from build123d import *

# Parameters (mm, degrees)
SKETCH1_W           = 20.828
SKETCH1_H           = 40.386
BOSS_EXTRUDE1_DEPTH = 38.1
SKETCH2_W           = 20.828
SKETCH2_H           = 59.8424
SKETCH2_R           = 1.98755
BOSS_EXTRUDE2_DEPTH = 2.6162
SKETCH5_R           = 2.8575
BOSS_EXTRUDE3_DEPTH = 4.2418
CHAMFER1_SIZE       = 5.08
FILLET4_R           = 1.016


with BuildPart() as part:
    # Sketch1 → Boss-Extrude1 (new body)
    with BuildSketch(Plane(origin=(0, 0, 0), x_dir=(1, 0, 0), z_dir=(0, 1, 0))):
        with Locations((10.414, 20.193)):
            Rectangle(SKETCH1_W, SKETCH1_H)
    extrude(amount=BOSS_EXTRUDE1_DEPTH)

    # Sketch2 → Boss-Extrude2 (add)
    with BuildSketch(Plane(origin=(0, 27.7368, 0), x_dir=(1, 0, 0), z_dir=(0, 1, 0))):
        with Locations((10.414, 20.193)):
            Rectangle(SKETCH2_W, SKETCH2_H)
        with Locations((4.8641, 45.2501)):
            Circle(SKETCH2_R, mode=Mode.SUBTRACT)
        with Locations((15.9639, 45.2501)):
            Circle(SKETCH2_R, mode=Mode.SUBTRACT)
        with Locations((15.9639, -4.8641)):
            Circle(SKETCH2_R, mode=Mode.SUBTRACT)
        with Locations((4.8641, -4.8641)):
            Circle(SKETCH2_R, mode=Mode.SUBTRACT)
    extrude(amount=BOSS_EXTRUDE2_DEPTH)

    # Sketch4 → Revolve1 (revolve)
    with BuildSketch(Plane(origin=(10.414, 0, 0), x_dir=(0, 0, -1), z_dir=(1, 0, 0))):
        Polygon((30.3911, 40.259), (26.289, 40.259), (24.3078, 38.1), (30.3911, 38.1), align=None)
    revolve(axis=Axis((10.414, 40.259, -30.3911), (0, -1, 0)))

    # Sketch5 → Boss-Extrude3 (add)
    with BuildSketch(Plane(origin=(0, 40.259, 0), x_dir=(1, 0, 0), z_dir=(0, 1, 0))):
        with Locations((10.414, 30.3911)):
            Circle(SKETCH5_R)
    extrude(amount=BOSS_EXTRUDE3_DEPTH)

    # Chamfer1
    chamfer1_edges = [part.edges().sort_by_distance(p)[0] for p in [
        (10.414, 38.1, 0),
    ]]
    chamfer(chamfer1_edges, length=CHAMFER1_SIZE)

    # Fillet4
    fillet4_edges = [part.edges().sort_by_distance(p)[0] for p in [
        (10.414, 38.1, -40.386),
        (20.828, 38.1, -22.733),
        (0, 38.1, -22.733),
        (10.414, 38.1, -36.4744),
        (10.414, 38.1, -5.08),
        (20.828, 35.56, -2.54),
        (10.414, 33.02, 0),
        (0, 35.56, -2.54),
        (10.414, 0, -40.386),
        (0, 13.8684, -40.386),
        (0, 0, -20.193),
        (20.828, 0, -20.193),
        (10.414, 0, 0),
        (20.828, 13.8684, -40.386),
        (0, 13.8684, 0),
        (20.828, 13.8684, 0),
        (0, 34.2265, -40.386),
        (20.828, 34.2265, -40.386),
        (0, 29.0449, 9.7282),
        (20.828, 29.0449, 9.7282),
        (0, 29.0449, -50.1142),
        (20.828, 29.0449, -50.1142),
    ]]
    fillet(fillet4_edges, radius=FILLET4_R)


solid = part.part
Verification items for the finished model (mm, model axes). A direction names the side the tool comes from. Round coordinates to 2 decimals unless told otherwise and drop trailing zeros. Loops run counter-clockwise (first coordinate to the right, second up) from the corner with the lowest first, then second, coordinate; pieces in that order, holes last. Notation, with made-up numbers: (-31, 18) - (-14, 18) arc R23 cw to (-14, 41) - close; hole circle Ø6 at (-16, 68). An arc over 180 degrees is marked (long way). Answer in a Markdown table with one row per item. Add a question column.
Q1. Section check B-B on z = 4. Enter the section's corners in (x, y), plus the area to 3 significant figures.
Q2. Release check for a two-part mould opening along X. For faces 4 (the face through (17.86, 29.03, 4.27)), 5 (the face through (0, 19, -20)), 6 (the face through (20.828, 19, -20)), 7 (the face through (10, 14, -40.386)) record: pulls with the +X half, pulls with the -X half, needs draft (parallel to the pull), parting line crosses it, or undercut.
Q3. Section check C-C on z = -38. Enter the section's corners in (x, y).
Q4. Section check A-A on y = 14.5. Enter the section's corners in (x, z), plus the area to 3 significant figures.
Q5. Gauge pin test, flat ends, axial feed: pin 1 (12 mm diameter, centred on x = 6, z = 7, fed in from -Y); pin 2 (12 mm diameter, centred on x = 17, y = 8, fed in from +Z); pin 3 (4 mm diameter, centred on x = 4.5, z = -6, fed in from +Y); pin 4 (3.5 mm diameter, centred on x = 4.86, z = 4.86, fed in from -Y). Record the tip position at first contact, or that the pin passes through.
Q6. Section check D-D on x = 15.5. State how many separate pieces and enclosed holes the cut face has, plus the area to 3 significant figures.
Q7. Tool access check on faces 1 (the face through (10, 30.353, 5)), 2 (the face through (10, 34, -40.386)), 3 (the face through (10, 14, 0)). Record the directions out of +Z, -Z, +X, -X, +Y, -Y that give a thin tool (end or side, any length) a straight path to the whole face; none if there is none.
Q8. Material ranges on line 1 (X direction, y = 28, z = -44.5); line 2 (Z direction, x = 16, y = 31.5); line 3 (Y direction, x = 1.5, z = -44), recorded low to high.
Found:
| question | item | result |
|---|---|---|
| 1 | outline | (0, 27.74) - (3.07, 27.74) - (3.07, 30.35) - (0, 30.35) - close; (6.65, 27.74) - (14.17, 27.74) - (14.17, 30.35) - (6.65, 30.35) - close; (17.75, 27.74) - (20.83, 27.74) - (20.83, 30.35) - (17.75, 30.35) - close |
| 1 | area | 35.8 mm² |
| 2 | face 4 | undercut |
| 2 | face 5 | pulls with the -X half |
| 2 | face 6 | pulls with the +X half |
| 2 | face 7 | needs draft |
| 3 | outline | (0, 1.02) arc R1.02 ccw to (1.02, 0) - (19.81, 0) arc R1.02 ccw to (20.83, 1.02) - (20.83, 37.08) arc R1.02 ccw to (19.81, 38.1) - (1.02, 38.1) arc R1.02 ccw to (0, 37.08) - close |
| 4 | outline | (0, -39.37) arc R1.02 ccw to (1.02, -40.39) - (19.81, -40.39) arc R1.02 ccw to (20.83, -39.37) - (20.83, -1.02) arc R1.02 ccw to (19.81, 0) - (1.02, 0) arc R1.02 ccw to (0, -1.02) - close |
| 4 | area | 840 mm² |
| 5 | pin 1 | stops at y = 27.74 |
| 5 | pin 2 | stops at z = 0 |
| 5 | pin 3 | stops at y = 38.1 |
| 5 | pin 4 | passes through |
| 6 | separate pieces | 3 |
| 6 | enclosed holes | 0 |
| 6 | area | 1,560 mm² |
| 7 | face 1 | +Z, +X, -X, +Y |
| 7 | face 2 | -Z, +X, -X, +Y |
| 7 | face 3 | +Z, +X, -X, -Y |
| 8 | line 1 | x = 0 to 3.02, 6.7 to 14.12, 17.8 to 20.83 |
| 8 | line 2 | z = -40.39 to 0 |
| 8 | line 3 | y = 27.74 to 30.35 |
